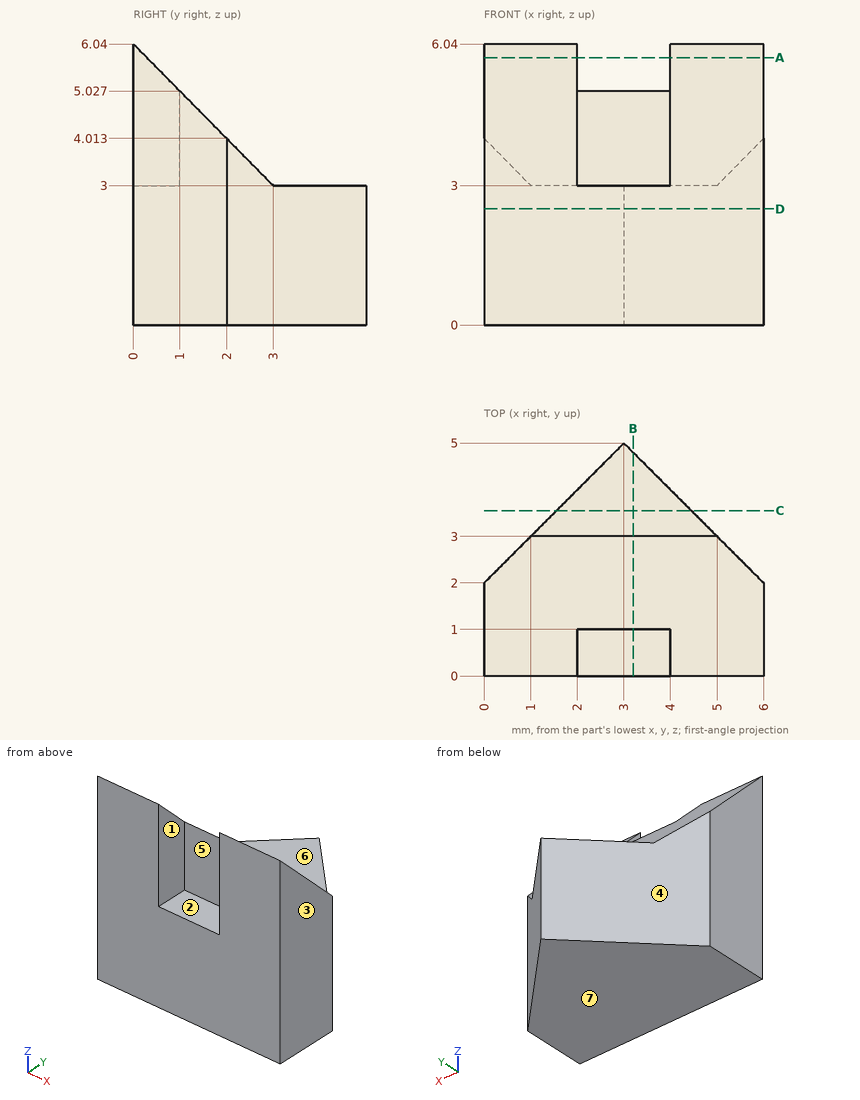
Study the drawing (mm; zero at the part's minimum x, y, z) and answer. A direction names the side the tool comes from. Round coordinates to 2 decimals unless told otherwise and drop trailing zeros. Write each loop counter-clockwise with the first axis right and the second up, starting at its lowest first coordinate (ties: lowest second). Pieces come first, ordered by that corner, then holes.
1) Determine the mould class of the marked faces 1, 2, 3 and 4 for opening direction X: pulls with the +X half, pulls with the -X half, needs draft (parallel to the pull), parting line crosses it, or undercut.
2) A cutting plane is placed at A-A on z = 5.75. Determine the outline of the cut face in (x, y).
3) Flat-ended cylindrical pins translate along their axes: P1, Ø2, axis at y = 4, z = 2, coming from the -X side; P2, Ø0.8, axis at x = 3, y = 0.5, coming from the +Z side; P3, Ø1, axis at x = 3, z = 4.5, coming from the -Y side. Find the tip coordinate at first contact, or state that the pin passes through.
4) Which of the six approach directions +Z, -Z, +X, -X, +Y, -Y give full straight-line access (tool end or side, diameter ignored) to the marked faces 5, 6 and 7?
5) Consider probe 1 along X at (y, z) = (0.45, 5); probe 2 along Y at (x, z) = (0.4, 1); probe 3 along Y at (x, z) = (5.05, 1.25). Determine where each line is inside the solid, lowest interval first.
6) A cutting plane is placed at B-B on x = 3.2. Determine the outline of the cut face in (y, z), and give its area (3 significant figures).
7) A cutting plane is placed at D-D on z = 2.5. Determine the outline of the cut face in (x, y).
8) A cutting plane is placed at C-C on y = 3.55. Determine the outline of the cut face in (x, z).
Entries:
1. face 1: undercut
1. face 2: undercut
1. face 3: pulls with the +X half
1. face 4: pulls with the -X half
2. outline: (0, 0) - (2, 0) - (2, 0.29) - (0, 0.29) - close; (4, 0) - (6, 0) - (6, 0.29) - (4, 0.29) - close
3. P1: stops at x = 1
3. P2: stops at z = 3
3. P3: stops at y = 1
4. face 5: +Z, -Y
4. face 6: +Z, +X, -X, +Y
4. face 7: -Z, +X, -X, +Y, -Y
5. probe 1: x = 0 to 2, 4 to 6
5. probe 2: y = 0 to 2.4
5. probe 3: y = 0 to 2.95
6. outline: (0, 0) - (4.8, 0) - (4.8, 3) - (3, 3) - (1, 5.03) - (1, 3) - (0, 3) - close
6. area: 16.4 mm2
7. outline: (0, 0) - (6, 0) - (6, 2) - (3, 5) - (0, 2) - close
8. outline: (1.55, 0) - (4.45, 0) - (4.45, 3) - (1.55, 3) - close
